from build123d import *

# Parameters (mm, degrees)
F1_DEPTH             = 60
F2_DEPTH             = 58
F9_D                 = 3.2
F9_DEPTH             = 4
F9_CSINK_D           = 6
F9_CSINK_ANGLE       = 90
F9_TIP               = 0.9613769904
F9_ON_F6_D           = 3.2
F9_ON_F6_DEPTH       = 4
F9_ON_F6_CSINK_D     = 6
F9_ON_F6_CSINK_ANGLE = 90
F9_ON_F6_TIP         = 0.9613769904
F9_ON_F8_D           = 3.2
F9_ON_F8_DEPTH       = 4
F9_ON_F8_CSINK_D     = 6
F9_ON_F8_CSINK_ANGLE = 90
F9_ON_F8_TIP         = 0.9613769904


# Not quite as in the source:
# - a feature names something its author has since deleted; it is built from what else it names


with BuildPart() as f1:
    # F0 (on Top) → F1 (new body)
    with BuildSketch(Plane.XY):
        with BuildLine():
            ThreePointArc((-13.375, -23.1661795512), (13.375, -23.1661795512), (26.75, 0))
            ThreePointArc((26.75, 0), (13.375, 23.1661795512), (-13.375, 23.1661795512))
            Line((-13.375, 23.1661795512), (-12.875, 22.3001541474))
            ThreePointArc((-12.875, 22.3001541474), (12.875, 22.3001541474), (25.75, 0))
            ThreePointArc((25.75, 0), (12.875, -22.3001541474), (-12.875, -22.3001541474))
            Line((-12.875, -22.3001541474), (-13.375, -23.1661795512))
        make_face()
        with BuildLine():
            Line((-12.875, 22.3001541474), (-13.375, 23.1661795512))
            ThreePointArc((-13.375, 23.1661795512), (-26.75, 0), (-13.375, -23.1661795512))
            Line((-13.375, -23.1661795512), (-12.875, -22.3001541474))
            ThreePointArc((-12.875, -22.3001541474), (-25.75, 0), (-12.875, 22.3001541474))
        make_face()
        with BuildLine():
            ThreePointArc((25.75, 0), (12.875, 22.3001541474), (-12.875, 22.3001541474))
            Line((-12.875, 22.3001541474), (0, 0))
            Line((0, 0), (-12.875, -22.3001541474))
            ThreePointArc((-12.875, -22.3001541474), (12.875, -22.3001541474), (25.75, 0))
        make_face()
        with BuildLine():
            Line((0, 0), (-12.875, 22.3001541474))
            ThreePointArc((-12.875, 22.3001541474), (-25.75, 0), (-12.875, -22.3001541474))
            Line((-12.875, -22.3001541474), (0, 0))
        make_face()
    extrude(amount=-F1_DEPTH)

    # F0 (on Top) → F2 (cut)
    with BuildSketch(Plane.XY):
        with BuildLine():
            ThreePointArc((25.75, 0), (12.875, 22.3001541474), (-12.875, 22.3001541474))
            Line((-12.875, 22.3001541474), (0, 0))
            Line((0, 0), (-12.875, -22.3001541474))
            ThreePointArc((-12.875, -22.3001541474), (12.875, -22.3001541474), (25.75, 0))
        make_face()
        with BuildLine():
            Line((0, 0), (-12.875, 22.3001541474))
            ThreePointArc((-12.875, 22.3001541474), (-25.75, 0), (-12.875, -22.3001541474))
            Line((-12.875, -22.3001541474), (0, 0))
        make_face()
    extrude(amount=-F2_DEPTH, mode=Mode.SUBTRACT)

    # F9
    with Locations(Plane(origin=(-13.375, 23.1661795512, 0), x_dir=(-0.8660254038, -0.5, 0), z_dir=(-0.5, 0.8660254038, 0))):
        with Locations((0, -5)):
            CounterSinkHole(F9_D / 2, F9_CSINK_D / 2, depth=F9_DEPTH, counter_sink_angle=F9_CSINK_ANGLE)
            with Locations((0, 0, -(F9_DEPTH + F9_TIP / 2))):  # 118° drill point
                Cone(0, F9_D / 2, F9_TIP, mode=Mode.SUBTRACT)

    # F9 on F6
    with Locations(Plane.YZ.offset(26.9)):
        with Locations((0, -5)):
            CounterSinkHole(F9_ON_F6_D / 2, F9_ON_F6_CSINK_D / 2, depth=F9_ON_F6_DEPTH, counter_sink_angle=F9_ON_F6_CSINK_ANGLE)
            with Locations((0, 0, -(F9_ON_F6_DEPTH + F9_ON_F6_TIP / 2))):  # 118° drill point
                Cone(0, F9_ON_F6_D / 2, F9_ON_F6_TIP, mode=Mode.SUBTRACT)

    # F9 on F8
    with Locations(Plane(origin=(-13.375, -23.1661795512, 0), x_dir=(0.8660254038, -0.5, 0), z_dir=(-0.5, -0.8660254038, 0))):
        with Locations((0, -5)):
            CounterSinkHole(F9_ON_F8_D / 2, F9_ON_F8_CSINK_D / 2, depth=F9_ON_F8_DEPTH, counter_sink_angle=F9_ON_F8_CSINK_ANGLE)
            with Locations((0, 0, -(F9_ON_F8_DEPTH + F9_ON_F8_TIP / 2))):  # 118° drill point
                Cone(0, F9_ON_F8_D / 2, F9_ON_F8_TIP, mode=Mode.SUBTRACT)


solid = f1.part
Part model, mm, in its own coordinate system. A direction names the side the tool comes from. Give positions to 0.01 mm unless a question says otherwise; leave off trailing zeros. Loops run counter-clockwise (first coordinate to the right, second up) from the corner with the lowest first, then second, coordinate; pieces in that order, holes last.
(1) Band-saw the part on D-D (x = 5). Write the cut outline in (y, z).
Return value:
outline: (-26.28, -60) - (26.28, -60) - (26.28, 0) - (25.26, 0) - (25.26, -58) - (-25.26, -58) - (-25.26, 0) - (-26.28, 0) - close
(2) Band-saw the part on A-A (z = -40.5). Write the cut outline in (x, y) (3 decimals).
Return value:
outline: circle Ø53.5 at (0, 0); hole circle Ø51.5 at (0, 0)
(3) Band-saw the part on B-B (z = -5). Write the cut outline in (x, y), and give its area (3 significant figures).
Return value:
outline: (-15.77, -21.61) - (-14.51, -21.27) arc R25.75 cw to (-14.51, 21.27) - (-15.77, 21.61) arc R26.75 ccw to start; (-11.17, -23.2) - (-10.83, -24.46) arc R26.75 ccw to (26.61, -2.71) - (25.69, -1.79) arc R25.75 cw to start; (-11.17, 23.2) arc R25.75 cw to (25.69, 1.79) - (26.61, 2.71) arc R26.75 ccw to (-10.83, 24.46) - close
area: 151 mm2
(4) Drill centre lines: line 1 along Z through (x, y) = (-15, -3.5); line 2 along Y through (x, z) = (-9, -49.5); line 3 along X through (y, z) = (3, -52). Where is each one in solid material? Low to high.
Return value:
line 1: z = -60 to -58
line 2: y = -25.19 to -24.13, 24.13 to 25.19
line 3: x = -26.58 to -25.57, 25.57 to 26.58
(5) Band-saw the part on C-C (y = -20). Write the cut outline in (x, z), and give its area (3 significant figures).
Return value:
outline: (-17.76, -60) - (17.76, -60) - (17.76, 0) - (16.22, 0) - (16.22, -58) - (-16.22, -58) - (-16.22, 0) - (-17.76, 0) - close
area: 250 mm2
(6) Pin check, flat tips, straight feed: pin 1 (5 mm diameter, centred on x = -18, z = -47.5, fed in from +Y); pin 2 (2 mm diameter, centred on x = 18, y = 15, fed in from +Z); pin 3 (12 mm diameter, centred on x = 18, z = -27, fed in from -Y). Stop position of each tip, or through.
Return value:
pin 1: stops at y = 21.8
pin 2: stops at z = -58
pin 3: stops at y = -23.91
(7) 3-axis set-ups, long thin cutter, end or side, ignore diameter. For faces 1 (the flat face through (0, 0, -58)), 2 (the flat face through (0, 0, -60)): which of +Z, -Z, +X, -X, +Y, -Y reach the whole face in a straight line?
Return value:
face 1: +Z
face 2: -Z, +X, -X, +Y, -Y
